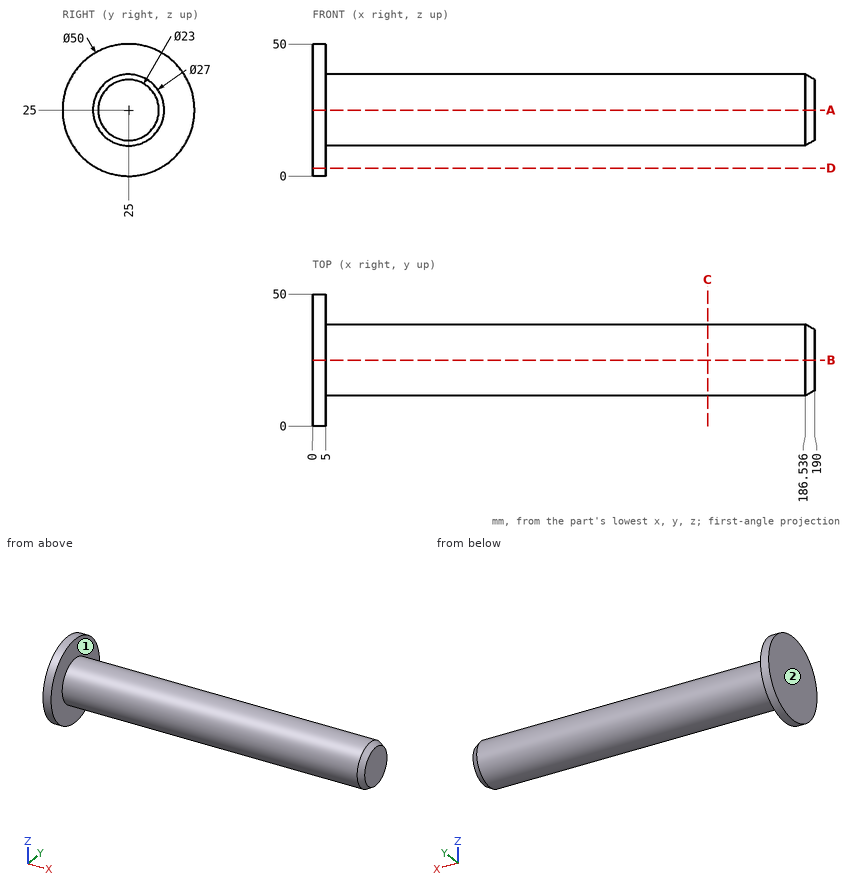
Geometry check sheet. Reference: drawing and pictorial views, mm from the part's lowest x, y, z. A direction names the side the tool comes from. Round coordinates to 2 decimals unless told otherwise and drop trailing zeros. Order: outer loops, then holes, each group sorted by start corner. A loop starts at its lowest first (then second) coordinate and runs counter-clockwise, first axis right, second up.
Q1. Depth check by flat-ended pin: P1, Ø1, axis at x = 49.5, y = 10.5, coming from the +Z side; P2, Ø8, axis at x = 80.5, y = 38, coming from the -Z side; P3, Ø12, axis at x = 76, z = 42.5, coming from the +Y side; P4, Ø12, axis at x = 76.5, z = 26.5, coming from the +Y side. Enter the tip coordinate at first touch or a pass-through.
Filled sheet:
P1: passes through
P2: stops at z = 14.94
P3: stops at y = 32.07
P4: stops at y = 38.5
Q2. Scan lines: L1, parallel to X at y = 15, z = 6; L2, parallel to X at y = 25.5, z = 13.5; L3, parallel to Z at x = 110.5, y = 26. Record each from-to range of solid material in increasing order.
Filled sheet:
L1: x = 0 to 5
L2: x = 0 to 189.98
L3: z = 11.54 to 38.46
Q3. Cross-section at A-A, the plane z = 25. Enter the section's corners in (x, y), plus the area to 3 significant figures.
Filled sheet:
outline: (0, 0) - (5, 0) - (5, 11.5) - (186.54, 11.5) - (190, 13.5) - (190, 36.5) - (186.54, 38.5) - (5, 38.5) - (5, 50) - (0, 50) - close
area: 5,240 mm2
Q4. Set-up check for the marked faces 1 and 2: record each of +Z, -Z, +X, -X, +Y, -Y from which the full face is reachable in a straight line by a thin tool's end or side.
Filled sheet:
face 1: +X
face 2: +Z, -Z, -X, +Y, -Y
Q5. Cross-section at C-C, the plane x = 149.5. Enter the section's corners in (y, z), plus the area to 3 significant figures.
Filled sheet:
outline: circle Ø27 at (25, 25)
area: 573 mm2
Q6. Cross-section at D-D, the plane z = 3. Enter the section's corners in (x, y).
Filled sheet:
outline: (0, 13.13) - (5, 13.13) - (5, 36.87) - (0, 36.87) - close
